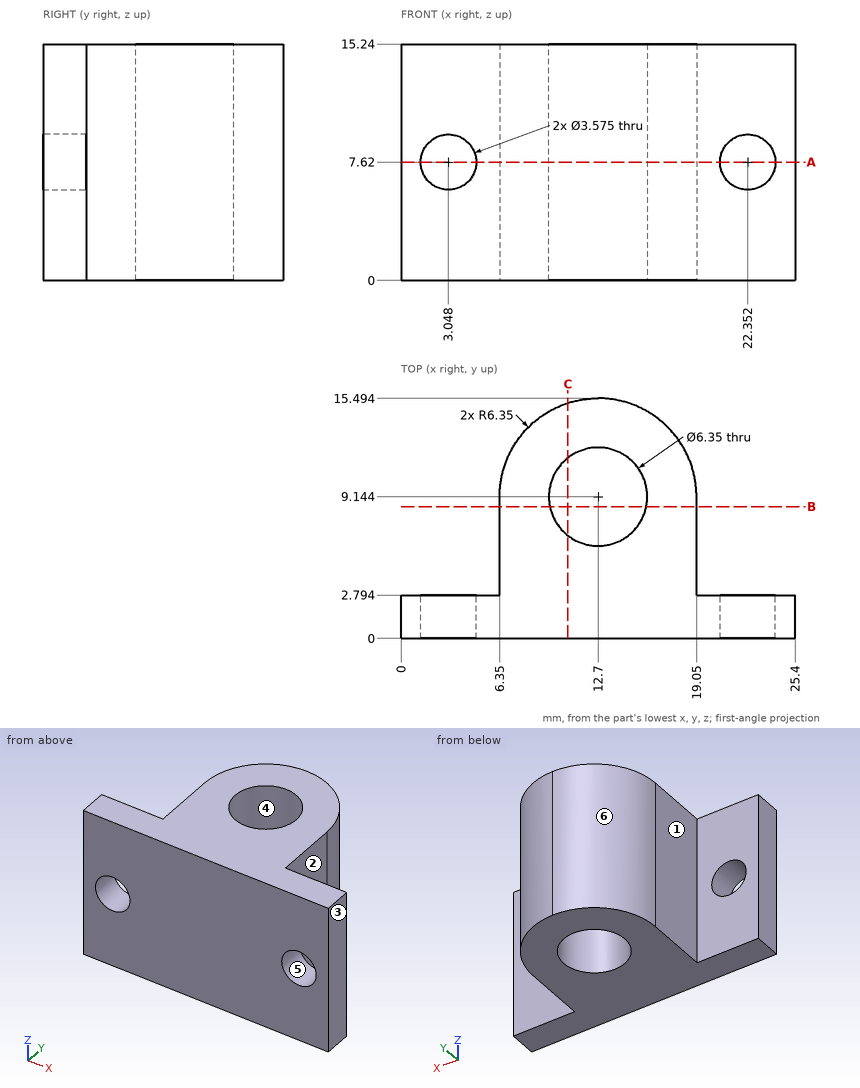
Verification items for this drawing (mm, ordinates from the low corner). A direction names the side the tool comes from. Give positions to 0.01 mm unless a question says otherwise; leave off trailing zeros. Loops run counter-clockwise (first coordinate to the right, second up) from the corner with the lowest first, then second, coordinate; pieces in that order, holes last. Notation, with made-up numbers: M 30.5,-36.75 L 60.5,-36.75 A18 cw 60.5,-26.75 Z; hole C 36,70.5 d3. An arc over 180 degrees is marked long. Answer as a JSON object with one key per item and string values. Group by question number.
Q1. Material ranges on line 1 along X through (y, z) = (0.6, 7.62); line 2 along Y through (x, z) = (12.7, 8.5); line 3 along Y through (x, z) = (5, 11.5), recorded low to high. Write a range as [from, to].
Q2. Access from +Z, -Z, +X, -X, +Y, -Y to the whole of each face (thin tool, end or side, straight path). Record for the marked faces 1, 2 and 3.
Q3. Cross-section at A-A on z = 7.62. Give the number of separate pieces and of enclosed holes in the cut face, then the cut area to 3 significant figures.
Q4. Go/stop test with flat-tipped pins: P1, Ø2, axis at x = 22.352, z = 7.62, coming from the +Y side; P2, Ø3, axis at x = 2, z = 10.5, coming from the +Y side; P3, Ø6, axis at x = 4.5, y = 9.5, coming from the +Z side; P4, Ø4, axis at y = 7.5, z = 8.5, coming from the +X side. Record where each tip stops, or that it passes through.
Q5. Release check for a two-part mould opening along Y. For the marked faces 4, 5 and 6 record: released by +Y, released by -Y, zero draft, split by the parting line, or undercut.
Q6. Cross-section at B-B on y = 8.5. Record the cut outline in (x, z).
Q7. Cross-section at C-C on x = 10.75. Record the cut outline in (y, z), then the cut area to 3 significant figures.
Evaluation:
{
 "1": {"line 1": "x = [0, 1.26], [4.84, 20.56], [24.14, 25.4]", "line 2": "y = [0, 5.97], [12.32, 15.49]", "line 3": "y = [0, 2.79]"},
 "2": {"face 1": "+Z, -Z, -X, +Y", "face 2": "+Z, -Z, +X, +Y", "face 3": "+Z, -Z, +X, +Y, -Y"},
 "3": {"separate pieces": "3", "enclosed holes": "1", "area": "163 mm2"},
 "4": {"P1": "passes through", "P2": "stops at y = 2.79", "P3": "stops at z = 15.24", "P4": "stops at x = 19.05"},
 "5": {"face 4": "undercut", "face 5": "zero draft", "face 6": "released by +Y"},
 "6": {"outline": "M 6.35,0 L 9.59,0 L 9.59,15.24 L 6.35,15.24 Z; M 15.81,0 L 19.05,0 L 19.05,15.24 L 15.81,15.24 Z"},
 "7": {"outline": "M 0,0 L 6.64,0 L 6.64,15.24 L 0,15.24 Z; M 11.65,0 L 15.19,0 L 15.19,15.24 L 11.65,15.24 Z", "area": "155 mm2"}
}
